Part print with two shaded views. Sizes in mm from the minimum x, y, z corner. A direction names the side the tool comes from. Coordinates: 2 decimals unless noted, no trailing zeros. Write each loop counter-clockwise with the first axis right and the second up, starting at its lowest first coordinate (ties: lowest second). Pieces come first, ordered by that corner, then holes. Notation, with made-up numbers: M 81,-40 L 123,-40 A30 cw 123,-9 Z; hole C 68.25,46 d8. An arc over 180 degrees is marked long. One line per question, with ' | ' between items. Start each with the question number.
(1) Wall check: probe 1 along X at (y, z) = (13.25, 12.7); probe 2 along Y at (x, z) = (25.5, 1.5) (3 decimals); probe 3 along Z at (x, y) = (23, 10.5). Give the ranges that are in metal, low to high.
(2) Flat gauge pins, fed straight in: pin 1 Ø6 at (x, z) = (13.5, 21.5) entering from -Y (3 decimals); pin 2 Ø5 at (y, z) = (3.5, 9) entering from +X. Where does each tip first touch, or does it go through?
(3) Two-plate mould, pull along X, no slides. Class the marked faces 1, 2 and 3: +X half, -X half, draft (parallel to the pull), parting line (faces both ways), or undercut.
(4) Tool access for the marked faces 4 and 5: list every direction of +Z, -Z, +X, -X, +Y, -Y with a clear straight run to the whole face (end or side of a thin tool).
(5) Cut at A-A (x = 5.08). Write the cut outline in (y, z) (3 decimals).
(6) Cut at C-C (y = 17.25). Write the cut outline in (x, z) (1 decimal), plus the area to 3 significant figures.
(7) Cut at D-D (x = 21). Write the cut outline in (y, z) (3 decimals), plus the area to 3 significant figures.
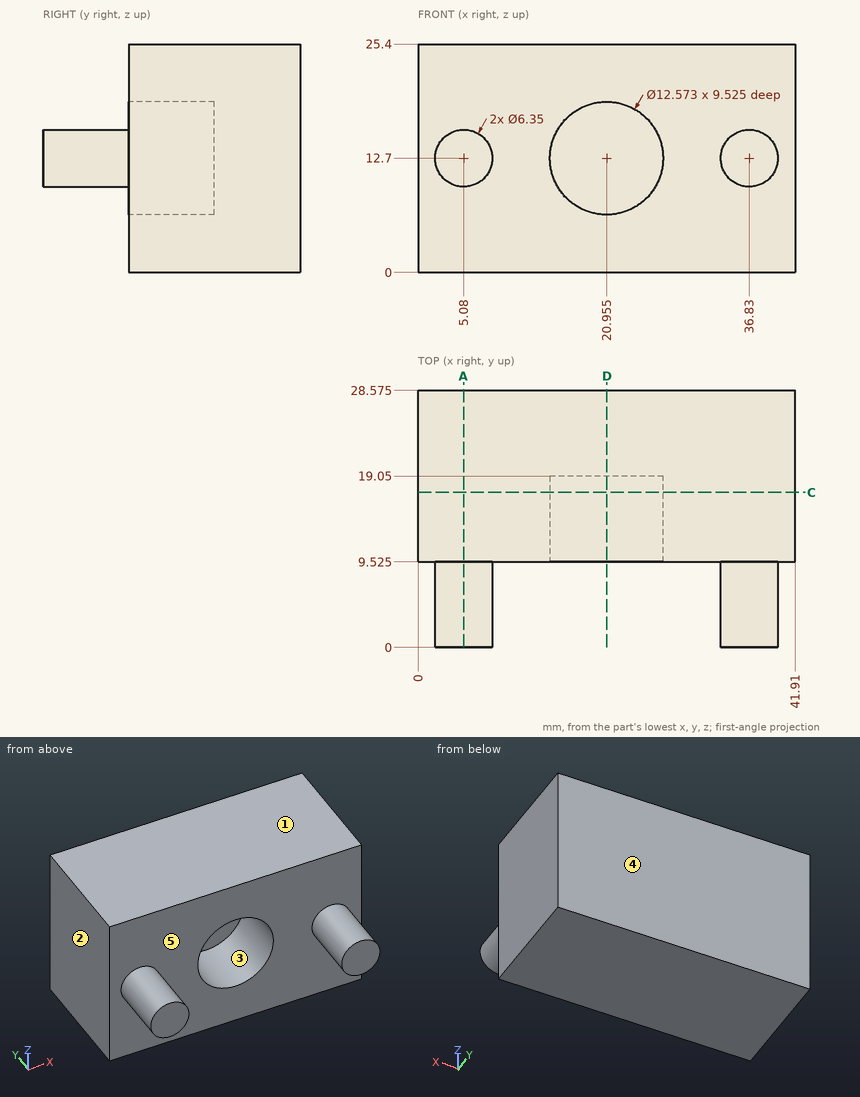
Filled in:
1) probe 1: 0 to 14.67, 27.24 to 41.91 | probe 2: 9.525 to 28.575 | probe 3: 0 to 6.76, 18.64 to 25.4
2) pin 1: y = 9.525 | pin 2: x = 39.77
3) face 1: draft | face 2: -X half | face 3: undercut
4) face 4: +Z, -Z, +X, -X, +Y | face 5: -Y
5) outline: M 0,9.525 L 9.525,9.525 L 9.525,0 L 28.575,0 L 28.575,25.4 L 9.525,25.4 L 9.525,15.875 L 0,15.875 Z
6) outline: M 0,0 L 41.9,0 L 41.9,25.4 L 0,25.4 Z; hole C 21,12.7 d12.6 | area: 940 mm²
7) outline: M 9.525,0 L 28.575,0 L 28.575,25.4 L 9.525,25.4 L 9.525,18.986 L 19.05,18.986 L 19.05,6.414 L 9.525,6.414 Z | area: 364 mm²
